```python
from build123d import *

# Parameters (mm, degrees)
F0_R     = 12.7
F1_DEPTH = 7.62
F3_DEPTH = 5.08
F7_R     = 15.24
F8_DEPTH = 5.08


# Not quite as in the source:
# - a fillet or chamfer that OpenCascade refuses, or shapes differently, is made with other operations: its cross-section is extruded or revolved along the edge and cut away or added
# - the program builds the solid bodies; features that only make, move or delete a surface that nothing else refers to are left out


with BuildPart() as f1:
    # F0 (on Top) → F1 (new body)
    with BuildSketch(Plane.XY):
        Circle(F0_R)
    extrude(amount=F1_DEPTH)

    # F2: chamfer of 8.89 x 8.8590220811 on 1 edges, made by hand

    # F2_s1 → F2_t2 (revolve, cut)
    with BuildSketch(Plane.XZ):
        Polygon((12.7, -1.2390220811), (3.81, 7.62), (12.7, 7.62), align=None)
    revolve(axis=Axis((0, 0, 7.62), (0, 0, 1)), mode=Mode.SUBTRACT)

    # F3 (add): a face of the model
    f3_faces = [f1.faces().sort_by_distance(p)[0] for p in [
        (0, 0, 0),
    ]]
    extrude(f3_faces, amount=F3_DEPTH)

    # F7 (on face) → F8 (join)
    with BuildSketch(Plane(origin=(0, 0, -5.08), x_dir=(1, 0, 0), z_dir=(0, 0, -1))):
        Circle(F7_R)
    extrude(amount=F8_DEPTH)


solid = f1.part
```
Geometry check sheet. Reference: the model listing, model coordinates, mm. A direction names the side the tool comes from. Coordinates: 2 decimals unless noted, no trailing zeros. Order: outer loops, then holes, each group sorted by start corner. A loop starts at its lowest first (then second) coordinate and runs counter-clockwise, first axis right, second up. Notation, with made-up numbers: (-34.75, 83.5) - (-22.75, 83.5) arc R11 ccw to (-22.75, 87.5) - close; hole circle Ø8 at (-37.75, 85). An arc over 180 degrees is marked (long way). Answer in a Markdown table with one row per item. Add a question column.
1. Section check C-C (z = -3). Enter the section's corners in (x, y), plus the area to 3 significant figures.
2. Section check A-A (y = 0). Enter the section's corners in (x, z), plus the area to 3 significant figures.
3. Material ranges on L1, parallel to X at y = -0.5, z = -8; L2, parallel to Z at x = -13, y = 7; L3, parallel to Y at x = 10, z = -1.25, recorded low to high. Write a range as [from, to].
4. Gauge pin test, flat ends, axial feed: pin 1 Ø10 at (y, z) = (5, 5) entering from -X; pin 2 Ø3 at (x, z) = (-3, 2) entering from +Y; pin 3 Ø5 at (x, y) = (10, 2.5) entering from +Z; pin 4 Ø8 at (y, z) = (-2.5, -8) entering from +X. Record the tip position at first contact, or that the pin passes through.
5. Section check D-D (z = 3.25). Enter the section's corners in (x, y), plus the area to 3 significant figures.
6. Access from +Z, -Z, +X, -X, +Y, -Y to the whole of each face (thin tool, end or side, straight path). Record for faces 1 (the face through (-3.3, 14.88, -7.58)), 2 (the face through (-2.484, -11.184, -2.504)).
Data:
| question | item | result |
|---|---|---|
| 1 | outline | circle Ø22.91 at (0, 0) |
| 1 | area | 412 mm² |
| 2 | outline | (-15.24, -10.16) - (15.24, -10.16) - (15.24, -5.08) - (11.46, -5.08) - (11.46, 0) - (3.81, 7.62) - (-3.81, 7.62) - (-11.46, 0) - (-11.46, -5.08) - (-15.24, -5.08) - close |
| 2 | area | 388 mm² |
| 3 | L1 | x = [-15.23, 15.23] |
| 3 | L2 | z = [-10.16, -5.08] |
| 3 | L3 | y = [-5.59, 5.59] |
| 4 | pin 1 | stops at x = -10.67 |
| 4 | pin 2 | stops at y = 10.59 |
| 4 | pin 3 | stops at z = 3.64 |
| 4 | pin 4 | stops at x = 15.24 |
| 5 | outline | circle Ø16.39 at (0, 0) |
| 5 | area | 211 mm² |
| 6 | face 1 | +Z, -Z |
| 6 | face 2 | +Z |
